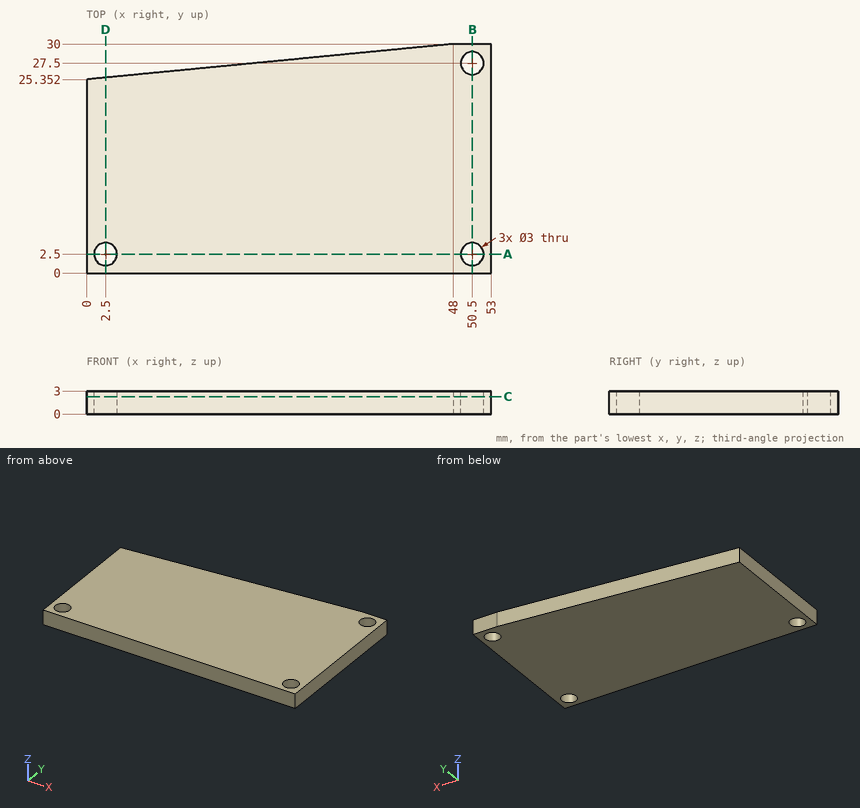
Could you check a few things on this drawing? It's one solid part, dimensions in mm from its lowest x, y, z. Round coordinates to 2 decimals unless told otherwise and drop trailing zeros. Write each loop counter-clockwise with the first axis right and the second up, starting at its lowest first coordinate (ties: lowest second). Pieces come first, ordered by that corner, then holes. Notation, with made-up numbers: (7.5, 82.5) -> (35.5, 82.5) arc R23 ccw to (35.5, 100.5) -> close; hole circle Ø9 at (54, 63.5). An arc over 180 degrees is marked (long way). Use a Markdown table: item, result.
1. If we section it at B-B (x = 50.5): List the corners of the cut face in (y, z) for me, then the cut area to 3 significant figures.
Answer key:
| item | result |
|---|---|
| outline | (0, 0) -> (1, 0) -> (1, 3) -> (0, 3) -> close; (4, 0) -> (26, 0) -> (26, 3) -> (4, 3) -> close; (29, 0) -> (30, 0) -> (30, 3) -> (29, 3) -> close |
| area | 72.0 mm^2 |
2. If we section it at C-C (z = 2.3): List the corners of the cut face in (x, y) for me.
Answer key:
| item | result |
|---|---|
| outline | (0, 0) -> (53, 0) -> (53, 30) -> (48, 30) -> (0, 25.35) -> close; hole circle Ø3 at (2.5, 2.5); hole circle Ø3 at (50.5, 2.5); hole circle Ø3 at (50.5, 27.5) |
3. If we section it at D-D (x = 2.5): List the corners of the cut face in (y, z) for me.
Answer key:
| item | result |
|---|---|
| outline | (0, 0) -> (1, 0) -> (1, 3) -> (0, 3) -> close; (4, 0) -> (25.59, 0) -> (25.59, 3) -> (4, 3) -> close |
4. Please list where these lines run through material, in increasing order: probe 1 along X at (y, z) = (2.5, 1); probe 2 along Y at (x, z) = (16, 2.85); probe 3 along Y at (x, z) = (40, 0.65).
Answer key:
| item | result |
|---|---|
| probe 1 | x = 0 to 1, 4 to 49, 52 to 53 |
| probe 2 | y = 0 to 26.9 |
| probe 3 | y = 0 to 29.23 |
5. If we section it at A-A (y = 2.5): List the corners of the cut face in (x, z) for me.
Answer key:
| item | result |
|---|---|
| outline | (0, 0) -> (1, 0) -> (1, 3) -> (0, 3) -> close; (4, 0) -> (49, 0) -> (49, 3) -> (4, 3) -> close; (52, 0) -> (53, 0) -> (53, 3) -> (52, 3) -> close |
